Can you work these out from the model? Positions are in its coordinate system, mm. A direction names the side the tool comes from. Coordinates: 2 decimals unless noted, no trailing zeros. Order: outer loops, then holes, each group sorted by start corner. A loop starts at its lowest first (then second) coordinate and runs counter-clockwise, first axis right, second up. Notation, with made-up numbers: (54.5, 1) -> (104.5, 1) arc R24 ccw to (104.5, 39) -> close; hole circle Ø11 at (35.5, -35.5). An arc over 180 degrees is marked (long way). Use a Markdown table: item, result. Add a question column.
1. Suppose I cut it at D-D, the plane z = 3.25. List the corners of the cut face in (x, y) for me, then the cut area to 3 significant figures.
2. For faces 4 (the cylindrical face through (0.878, -0.822, -3.954)), 5 (the cylindrical face through (5, 6, 0)), which set-ups out of +Z, -Z, +X, -X, +Y, -Y let a thin tool reach every point of the face, with its end or its side?
3. Suppose I cut it at C-C, the plane y = 4.5. List the corners of the cut face in (x, z) for me, then the cut area to 3 significant figures.
4. If I drill on line 1 along Z through (x, y) = (0, 5.05); line 2 along Z through (x, y) = (0, 1.75); line 3 along Y through (x, z) = (4, 3.25), over which ranges is the centre line in solid material (lowest first)? Write a range as from..to.
5. We'd pull the mould along Z, two halves only. Please class faces 1 (the flat face through (-2, 2.573, 5)), 2 (the cylindrical face through (5, -3, 0)), 3 (the cylindrical face through (-0.81, 4.09, -9.3)): pulls with the +Z half, pulls with the -Z half, needs draft (parallel to the pull), parting line crosses it, or undercut.
6. Suppose I cut it at A-A, the plane z = 0. List the corners of the cut face in (x, y) for me.
7. For pin 1 Ø6 at (x, z) = (7.5, 3) entering from +Y; pin 2 Ø7.5 at (x, z) = (0, 0) entering from +Y; pin 3 Ø1.5 at (x, y) = (-2.5, -4.5) entering from -Z; pin 4 Ø6 at (x, y) = (-1.5, 3.5) entering from -Z, each with a flat end and sliding along its axis, tell me the tip position at first contact or that it passes through.
8. Suppose I cut it at B-B, the plane x = 0. List the corners of the cut face in (y, z) for me, then the cut area to 3 significant figures.
```python
from build123d import *

# Parameters (mm, degrees)
KES_EKSTR_ZYON1_REACH = 23.61
IZIM2_R               = 4.05
KES_EKSTR_ZYON2_REACH = 22.928
IZIM3_R               = 1.75


with BuildPart() as part:
    # Çizim1 → Döndür1 (revolve)
    with BuildSketch(Plane.XY, mode=Mode.PRIVATE) as d_nd_r1_sk:
        Polygon((0, 6.572949203), (5, 6.572949203), (5, 5.572949203), (11, 5.572949203), (11, 2.572949203), (5, 2.572949203), (5, -8.427050797), (0, -8.427050797), align=None)
    revolve(d_nd_r1_sk.sketch.rotate(Axis((0, 6.572949203, 0), (0, -1, 0)), 180), axis=Axis((0, 6.572949203, 0), (0, -1, 0)))

    # Çizim2 → Kes-Ekstrüzyon1 (cut, up to next)
    with BuildSketch(Plane(origin=(0, 6.572949203, 0), x_dir=(1, 0, 0), z_dir=(0, 1, 0)), mode=Mode.PRIVATE) as kes_ekstr_zyon1_sk1:
        with Locations(Location((0, 0, 0), (0, 0, 180))):
            Circle(IZIM2_R)
    kes_ekstr_zyon1_tool1 = extrude(kes_ekstr_zyon1_sk1.sketch, amount=-KES_EKSTR_ZYON1_REACH, mode=Mode.PRIVATE) & part.part
    add(kes_ekstr_zyon1_tool1.solids().sort_by_distance((0, 6.572949, 0))[0], mode=Mode.SUBTRACT)

    # Çizim3 → Kes-Ekstrüzyon2 (cut, up to next)
    with BuildSketch(Plane(origin=(0, 5.572949203, 0), x_dir=(1, 0, 0), z_dir=(0, 1, 0)), mode=Mode.PRIVATE) as kes_ekstr_zyon2_sk1:
        with Locations(Location((0, 7.75, 0), (0, 0, 180))):
            Circle(IZIM3_R)
    kes_ekstr_zyon2_tool1 = extrude(kes_ekstr_zyon2_sk1.sketch, amount=-KES_EKSTR_ZYON2_REACH, mode=Mode.PRIVATE) & part.part
    # Çizim3 → Kes-Ekstrüzyon2 (cut, up to next)
    with BuildSketch(Plane(origin=(0, 5.572949203, 0), x_dir=(1, 0, 0), z_dir=(0, 1, 0)), mode=Mode.PRIVATE) as kes_ekstr_zyon2_sk2:
        with Locations(Location((7.75, 0, 0), (0, 0, 180))):
            Circle(IZIM3_R)
    kes_ekstr_zyon2_tool2 = extrude(kes_ekstr_zyon2_sk2.sketch, amount=-KES_EKSTR_ZYON2_REACH, mode=Mode.PRIVATE) & part.part
    # Çizim3 → Kes-Ekstrüzyon2 (cut, up to next)
    with BuildSketch(Plane(origin=(0, 5.572949203, 0), x_dir=(1, 0, 0), z_dir=(0, 1, 0)), mode=Mode.PRIVATE) as kes_ekstr_zyon2_sk3:
        with Locations(Location((0, -7.75, 0), (0, 0, 180))):
            Circle(IZIM3_R)
    kes_ekstr_zyon2_tool3 = extrude(kes_ekstr_zyon2_sk3.sketch, amount=-KES_EKSTR_ZYON2_REACH, mode=Mode.PRIVATE) & part.part
    # Çizim3 → Kes-Ekstrüzyon2 (cut, up to next)
    with BuildSketch(Plane(origin=(0, 5.572949203, 0), x_dir=(1, 0, 0), z_dir=(0, 1, 0)), mode=Mode.PRIVATE) as kes_ekstr_zyon2_sk4:
        with Locations(Location((-7.75, 0, 0), (0, 0, 180))):
            Circle(IZIM3_R)
    kes_ekstr_zyon2_tool4 = extrude(kes_ekstr_zyon2_sk4.sketch, amount=-KES_EKSTR_ZYON2_REACH, mode=Mode.PRIVATE) & part.part
    add(kes_ekstr_zyon2_tool1.solids().sort_by_distance((0, 5.572949, -7.75))[0], mode=Mode.SUBTRACT)
    add(kes_ekstr_zyon2_tool2.solids().sort_by_distance((7.75, 5.572949, 0))[0], mode=Mode.SUBTRACT)
    add(kes_ekstr_zyon2_tool3.solids().sort_by_distance((0, 5.572949, 7.75))[0], mode=Mode.SUBTRACT)
    add(kes_ekstr_zyon2_tool4.solids().sort_by_distance((-7.75, 5.572949, 0))[0], mode=Mode.SUBTRACT)


solid = part.part
```
Worked out:
| question | item | result |
|---|---|---|
| 1 | outline | (-10.51, 2.57) -> (-3.8, 2.57) -> (-3.8, -8.43) -> (-2.42, -8.43) -> (-2.42, 6.57) -> (-3.8, 6.57) -> (-3.8, 5.57) -> (-10.51, 5.57) -> close; (2.42, -8.43) -> (3.8, -8.43) -> (3.8, 2.57) -> (10.51, 2.57) -> (10.51, 5.57) -> (3.8, 5.57) -> (3.8, 6.57) -> (2.42, 6.57) -> close |
| 1 | area | 81.7 mm² |
| 2 | face 4 | +Y, -Y |
| 2 | face 5 | +Y |
| 3 | outline | circle Ø22 at (0, 0); hole circle Ø3.5 at (-7.75, 0); hole circle Ø8.1 at (0, 0); hole circle Ø3.5 at (0, -7.75); hole circle Ø3.5 at (0, 7.75); hole circle Ø3.5 at (7.75, 0) |
| 3 | area | 290 mm² |
| 4 | line 1 | z = -11..-9.5, -6..-4.05, 4.05..6, 9.5..11 |
| 4 | line 2 | z = -5..-4.05, 4.05..5 |
| 4 | line 3 | y = 2.57..5.57 |
| 5 | face 1 | needs draft |
| 5 | face 2 | parting line crosses it |
| 5 | face 3 | undercut |
| 6 | outline | (-11, 2.57) -> (-9.5, 2.57) -> (-9.5, 5.57) -> (-11, 5.57) -> close; (-6, 2.57) -> (-5, 2.57) -> (-5, -8.43) -> (-4.05, -8.43) -> (-4.05, 6.57) -> (-5, 6.57) -> (-5, 5.57) -> (-6, 5.57) -> close; (4.05, -8.43) -> (5, -8.43) -> (5, 2.57) -> (6, 2.57) -> (6, 5.57) -> (5, 5.57) -> (5, 6.57) -> (4.05, 6.57) -> close; (9.5, 2.57) -> (11, 2.57) -> (11, 5.57) -> (9.5, 5.57) -> close |
| 7 | pin 1 | stops at y = 5.57 |
| 7 | pin 2 | passes through |
| 7 | pin 3 | stops at z = -4.68 |
| 7 | pin 4 | stops at z = -11 |
| 8 | outline | (-8.43, -5) -> (2.57, -5) -> (2.57, -6) -> (5.57, -6) -> (5.57, -5) -> (6.57, -5) -> (6.57, -4.05) -> (-8.43, -4.05) -> close; (-8.43, 4.05) -> (6.57, 4.05) -> (6.57, 5) -> (5.57, 5) -> (5.57, 6) -> (2.57, 6) -> (2.57, 5) -> (-8.43, 5) -> close; (2.57, -11) -> (5.57, -11) -> (5.57, -9.5) -> (2.57, -9.5) -> close; (2.57, 9.5) -> (5.57, 9.5) -> (5.57, 11) -> (2.57, 11) -> close |
| 8 | area | 43.5 mm² |
